Here's the drawing with two shaded views (mm, measured from the low corner). I have some questions. A direction names the side the tool comes from. Round coordinates to 2 decimals unless told otherwise and drop trailing zeros. Loops run counter-clockwise (first coordinate to the right, second up) from the corner with the lowest first, then second, coordinate; pieces in that order, holes last. Notation, with made-up numbers: M 24,15.25 L 39,15.25 A27 ccw 39,48.25 Z; hole C 64.5,32 d8. An arc over 180 degrees is marked long. Answer as a JSON object with one key per item and string values.
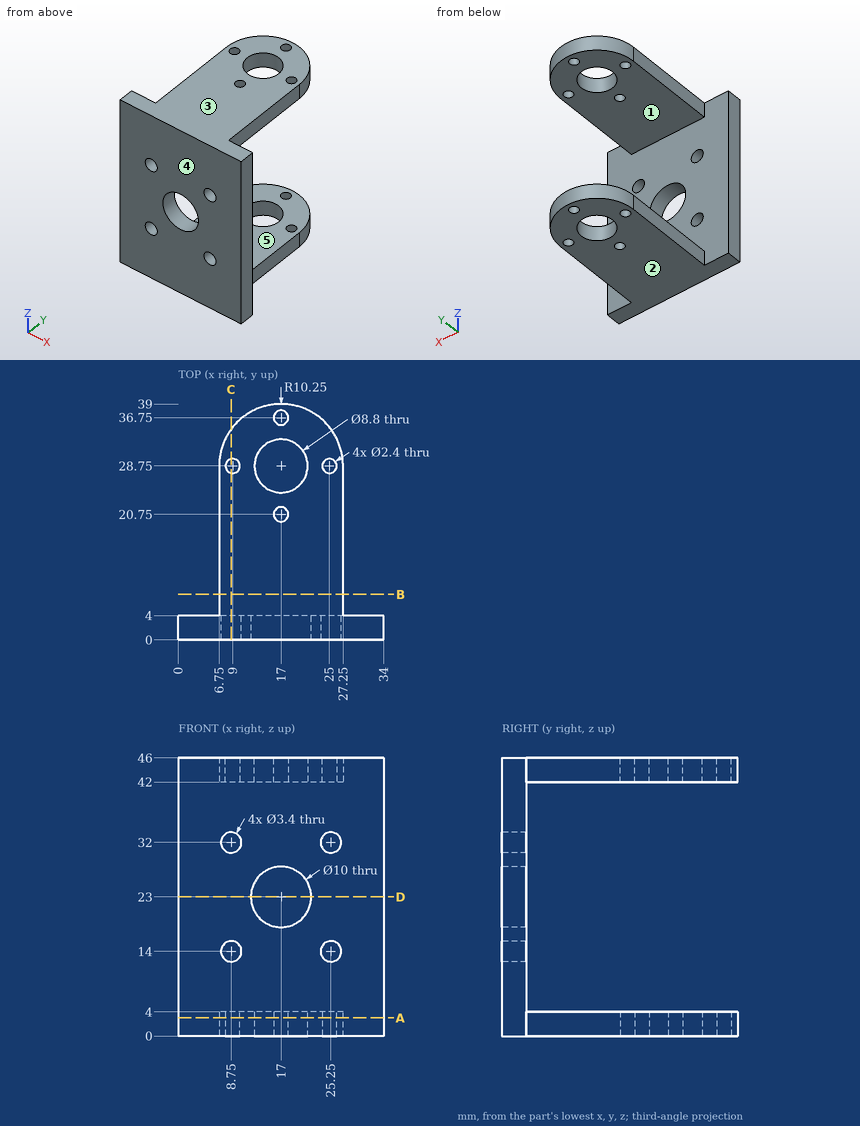
Item 1: I want a section at C-C on x = 8.75. List the corners of the cut face in (y, z) for me, plus the area to 3 significant figures.
Solution:
{"outline": "M 0,0 L 27.58,0 L 27.58,4 L 4,4 L 4,12.3 L 0,12.3 Z; M 0,15.7 L 4,15.7 L 4,30.3 L 0,30.3 Z; M 0,33.7 L 4,33.7 L 4,42 L 27.58,42 L 27.58,46 L 0,46 Z; M 29.92,0 L 34.83,0 L 34.83,4 L 29.92,4 Z; M 29.92,42 L 34.83,42 L 34.83,46 L 29.92,46 Z", "area": "385 mm2"}
Item 2: I want a section at D-D on z = 23. List the corners of the cut face in (x, y) for me.
Solution:
{"outline": "M 0,0 L 12,0 L 12,4 L 0,4 Z; M 22,0 L 34,0 L 34,4 L 22,4 Z"}
Item 3: If I drill on L1, parallel to Z at x = 8.75, y = 1.8; L2, parallel to Y at x = 17, z = 3.25; L3, parallel to Z at x = 20, y = 22.5, over which ranges is the centre line in solid material (lowest first)? Write a range as from..to.
Solution:
{"L1": "z = 0..12.3, 15.7..30.3, 33.7..46", "L2": "y = 0..19.55, 21.95..24.35, 33.15..35.55, 37.95..39", "L3": "z = 0..4, 42..46"}
Item 4: I want a section at A-A on z = 3. List the corners of the cut face in (x, y) for me, plus the area to 3 significant figures.
Solution:
{"outline": "M 0,0 L 34,0 L 34,4 L 27.25,4 L 27.25,28.75 A10.25 ccw 6.75,28.75 L 6.75,4 L 0,4 Z; hole C 9,28.75 d2.4; hole C 17,28.75 d8.8; hole C 17,20.75 d2.4; hole C 17,36.75 d2.4; hole C 25,28.75 d2.4", "area": "729 mm2"}
Item 5: For the marked faces 1 and 2, which set-ups out of +Z, -Z, +X, -X, +Y, -Y let a thin tool reach every point of the face, with its end or its side?
Solution:
{"face 1": "+X, -X, +Y", "face 2": "-Z, +X, -X, +Y, -Y"}
Item 6: We'd pull the mould along Z, two halves only. Please class the marked faces 3, 4 and 5: +Z half, -Z half, draft (parallel to the pull), parting line (faces both ways), or undercut.
Solution:
{"face 3": "+Z half", "face 4": "draft", "face 5": "undercut"}
Item 7: For P1, Ø12, axis at x = 9.5, z = 5.5, coming from the +Y side; P2, Ø2, axis at x = 17, y = 36.75, coming from the +Z side; P3, Ø1.2, axis at y = 15.5, z = 1, coming from the -X side; P4, Ø2, axis at y = 13, z = 2, coming from the +X side, each with a flat end and sliding along its axis, tell me the tip position at first contact or that it passes through.
Solution:
{"P1": "stops at y = 38.86", "P2": "passes through", "P3": "stops at x = 6.75", "P4": "stops at x = 27.25"}
Item 8: I want a section at B-B on y = 7.5. List the corners of the cut face in (x, z) for me, plus the area to 3 significant figures.
Solution:
{"outline": "M 6.75,0 L 27.25,0 L 27.25,4 L 6.75,4 Z; M 6.75,42 L 27.25,42 L 27.25,46 L 6.75,46 Z", "area": "164 mm2"}
